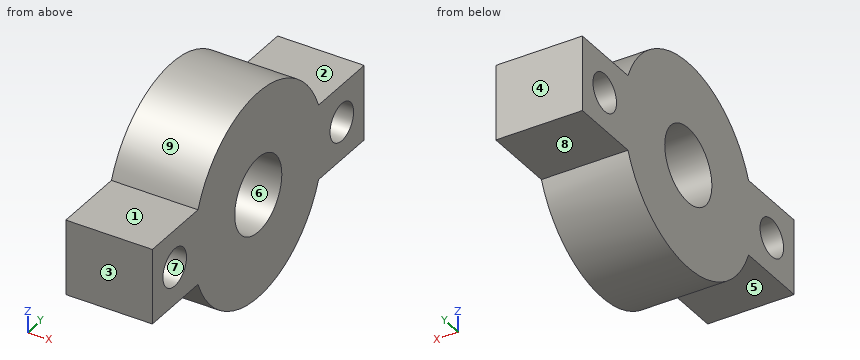
Autodesk Inventor part; units mm, degrees
ref_plane "YZ Plane" through (0, 0, 0) normal (1, 0, 0) x (0, 1, 0)
ref_plane "XZ Plane" through (0, 0, 0) normal (0, 1, 0) x (-1, 0, 0)
ref_plane "XY Plane" through (0, 0, 0) normal (0, 0, 1) x (1, 0, 0)
sketch "Sketch1" plane through (0, 0, 0) normal (1, 0, 0) x (0, 1, 0)
  circle A0 centre (0, 0) radius 10
  circle A1 centre (0, 0) radius 27.5
  circle A2 centre (35.5, 0) radius 5
  circle A3 centre (-35.5, 0) radius 5
  line L0 (-35.5, 0) -> (35.5, 0) construction
  line L1 (0, 0) -> (10, 0) construction
  line L2 (0, 0) -> (10, 0) construction
  line L3 (-45, 10) -> (45, 10)
  line L4 (45, 10) -> (45, -10)
  line L5 (45, -10) -> (-45, -10)
  line L6 (-45, -10) -> (-45, 10)
  line L7 (-45, 10) -> (45, -10) construction
  line L8 (45, 10) -> (-45, -10) construction
  dimension "d0" = 20
  dimension "d1" = 55
  dimension "d2" = 10
  dimension "d3" = 10
  dimension "d4" = 71
  dimension "d5" = 10
  dimension "d6" = 0
  dimension "d7" = 35.5
  dimension "d8" = 90
  dimension "d9" = 20
extrude "Extrusion1" add sketch "Sketch1" along normal blind 23 contours A0 L3 A1 L5 | A0 L5 A1 L3 | L3 A1 | L5 A1 | A1 L5 L6 L3 | L3 L4 L5 A1
properties part number "KFL004"
The listing builds one solid part. Answer for the finished solid, in the listing's coordinates (mm). Face numbers are marked on the shaded views. A direction names the side the tool comes from. Round coordinates to 2 decimals unless told otherwise and drop trailing zeros. Write each loop counter-clockwise with the first axis right and the second up, starting at its lowest first coordinate (ties: lowest second). Pieces come first, ordered by that corner, then holes. Notation, with made-up numbers: M 27,50 L 31,50 A30 cw 31,72 Z; hole C 57.25,-19 d9. An arc over 180 degrees is marked long. Write each question's results on one line, items separated by ' | '. Start each with the question number.
Item 1: For a pull along Z with two mould halves and no side action, classify the marked faces 6, 7, 8 and 9 as pulls with the +Z half, pulls with the -Z half, needs draft (parallel to the pull), parting line crosses it, or undercut.
Item 2: Flat-ended cylindrical pins translate along their axes: pin 1 Ø9.5 at (x, y) = (13, 36) entering from -Z; pin 2 Ø1 at (x, y) = (11, 29.5) entering from +Z; pin 3 Ø1.5 at (x, y) = (3.5, -12.5) entering from +Z. Find the tip coordinate at first contact, or state that the pin passes through.
Item 3: A cutting plane is placed at A-A on y = 0. Write down the section's boundary in (x, z), and give its area (3 significant figures).
Item 4: For the marked faces 1, 2, 3, 4 and 5, determine the directions among +Z, -Z, +X, -X, +Y, -Y from which every point of the face is accessible in a straight line to the end or side of a thin tool.
Item 5: A cutting plane is placed at B-B on z = 0. Write down the section's boundary in (x, y), and give its area (3 significant figures).
Item 6: Straight lines are drawn through the part: L1, parallel to Z at x = 10.75, y = 35.5; L2, parallel to Y at x = 7.25, z = 4; L3, parallel to Y at x = 10.5, z = 3.5. For each, find the intervals that lie inside material, in ascending order. Write a range as [from, to].
Item 7: A cutting plane is placed at C-C on x = 7.5. Write down the section's boundary in (y, z), and give its area (3 significant figures).
Item 8: A cutting plane is placed at D-D on y = 35.5. Write down the section's boundary in (x, z), and give its area (3 significant figures).
Check sheet entries:
1) face 6: undercut | face 7: undercut | face 8: pulls with the -Z half | face 9: pulls with the +Z half
2) pin 1: z = -10 | pin 2: z = 10 | pin 3: z = 24.86
3) outline: M 0,-27.5 L 23,-27.5 L 23,-10 L 0,-10 Z; M 0,10 L 23,10 L 23,27.5 L 0,27.5 Z | area: 805 mm²
4) face 1: +Z, +X, -X, -Y | face 2: +Z, +X, -X, +Y | face 3: +Z, -Z, +X, -X, -Y | face 4: +Z, -Z, +X, -X, +Y | face 5: -Z, +X, -X, -Y
5) outline: M 0,-45 L 23,-45 L 23,-40.5 L 0,-40.5 Z; M 0,-30.5 L 23,-30.5 L 23,-10 L 0,-10 Z; M 0,10 L 23,10 L 23,30.5 L 0,30.5 Z; M 0,40.5 L 23,40.5 L 23,45 L 0,45 Z | area: 1,150 mm²
6) L1: [-10, -5], [5, 10] | L2: [-45, -38.5], [-32.5, -9.17], [9.17, 32.5], [38.5, 45] | L3: [-45, -39.07], [-31.93, -9.37], [9.37, 31.93], [39.07, 45]
7) outline: M -45,-10 L -25.62,-10 A27.5 ccw 25.62,-10 L 45,-10 L 45,10 L 25.62,10 A27.5 ccw -25.62,10 L -45,10 Z; hole C -35.5,0 d10; hole C 0,0 d20; hole C 35.5,0 d10 | area: 2,630 mm²
8) outline: M 0,-10 L 23,-10 L 23,-5 L 0,-5 Z; M 0,5 L 23,5 L 23,10 L 0,10 Z | area: 230 mm²
